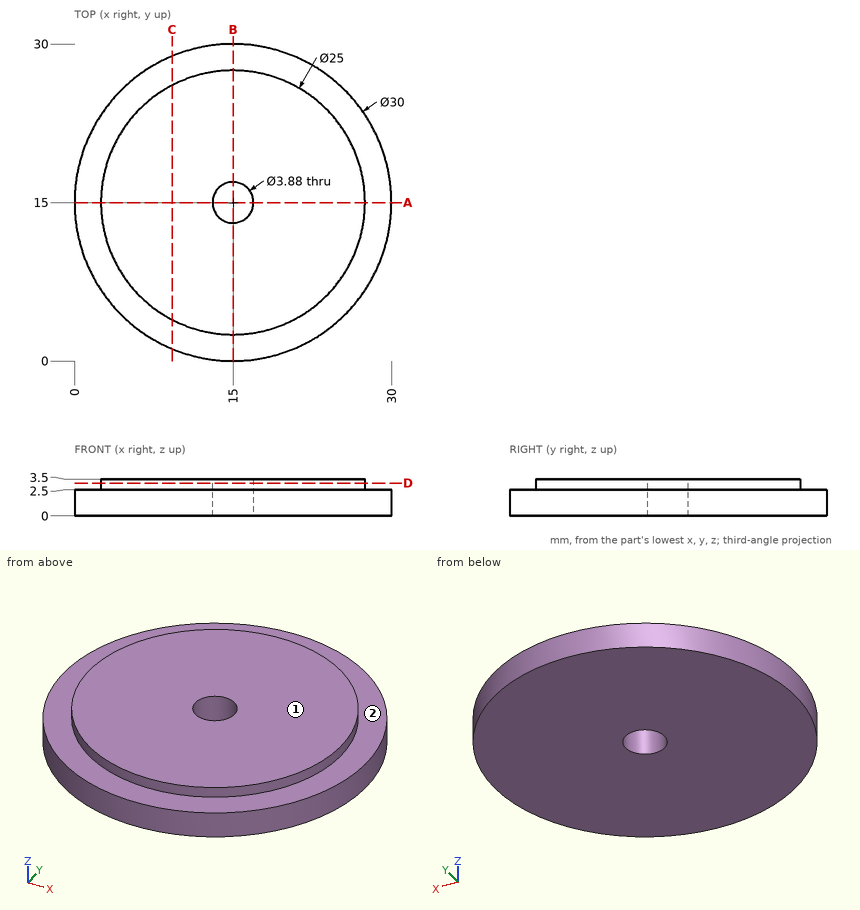
Here's the drawing with two shaded views (mm, measured from the low corner). I have some questions. A direction names the side the tool comes from. Round coordinates to 2 decimals unless told otherwise and drop trailing zeros. Order: outer loops, then holes, each group sorted by start corner. A loop starts at its lowest first (then second) coordinate and runs counter-clockwise, first axis right, second up. Notation, with made-up numbers: (33.25, 33.5) -> (47.25, 33.5) arc R12 cw to (47.25, 45.5) -> close; hole circle Ø2 at (66.5, 73.5). An arc over 180 degrees is marked (long way). Return JSON: item names as keys, results as strings.
Q1. If we section it at D-D on z = 3.1: List the corners of the cut face in (x, y) for me, plus the area to 3 significant figures.
Filled sheet:
{"outline": "circle Ø25 at (15, 15); hole circle Ø3.88 at (15, 15)", "area": "479 mm^2"}
Q2. If we section it at C-C on x = 9.25: List the corners of the cut face in (y, z) for me.
Filled sheet:
{"outline": "(1.15, 0) -> (28.85, 0) -> (28.85, 2.5) -> (26.1, 2.5) -> (26.1, 3.5) -> (3.9, 3.5) -> (3.9, 2.5) -> (1.15, 2.5) -> close"}
Q3. For pin 1 Ø1.5 at (x, z) = (8.5, 1) entering from -Y; pin 2 Ø1 at (y, z) = (8, 1.5) entering from +X; pin 3 Ø2 at (y, z) = (18, 1) entering from -X; pin 4 Ø3 at (x, y) = (15, 15) entering from -Z, each with a flat end and sliding along its axis, tell me the tip position at first contact or that it passes through.
Filled sheet:
{"pin 1": "stops at y = 1.15", "pin 2": "stops at x = 28.52", "pin 3": "stops at x = 0.13", "pin 4": "passes through"}
Q4. If we section it at A-A on y = 15: List the corners of the cut face in (x, z) for me, plus the area to 3 significant figures.
Filled sheet:
{"outline": "(0, 0) -> (13.06, 0) -> (13.06, 3.5) -> (2.5, 3.5) -> (2.5, 2.5) -> (0, 2.5) -> close; (16.94, 0) -> (30, 0) -> (30, 2.5) -> (27.5, 2.5) -> (27.5, 3.5) -> (16.94, 3.5) -> close", "area": "86.4 mm^2"}
Q5. Which directions (+Z, -Z, +X, -X, +Y, -Y) give clear straight access to the entire face, cutting with the end or side of a thin tool? Please do the marked faces 1 and 2.
Filled sheet:
{"face 1": "+Z, +X, -X, +Y, -Y", "face 2": "+Z"}
Q6. I need wall thicknesses on line 1 along Y through (x, z) = (15, 1.9); line 2 along Z through (x, y) = (7.5, 4); line 3 along X through (y, z) = (14.5, 0.9). Which ranges of each line are inside material? Lowest first, please. Write a range as from..to.
Filled sheet:
{"line 1": "y = 0..13.06, 16.94..30", "line 2": "z = 0..2.5", "line 3": "x = 0.01..13.13, 16.87..29.99"}
